from build123d import *

# Parameters (mm, degrees)
SKETCH1_W           = 88.9
SKETCH1_H           = 203.2
BOSS_EXTRUDE1_DEPTH = 6.35
SKETCH2_R           = 3
SKETCH2_R_2         = 2.75
SKETCH2_R_3         = 12.7
CUT_EXTRUDE1_DEPTH  = 7.35


with BuildPart() as part:
    # Sketch1 → Boss-Extrude1 (new body)
    with BuildSketch(Plane(origin=(0, 0, 0), x_dir=(1, 0, 0), z_dir=(0, 1, 0))):
        with Locations((44.45, 101.6)):
            Rectangle(SKETCH1_W, SKETCH1_H)
    extrude(amount=BOSS_EXTRUDE1_DEPTH)

    # Sketch2 → Cut-Extrude1 (cut, through all)
    with BuildSketch(Plane.XZ):
        with Locations((20.6375, -7.913544442)):
            Circle(SKETCH2_R)
        with Locations((68.2625, -7.913544442)):
            Circle(SKETCH2_R)
        with Locations((44.45, -112.75)):
            Circle(SKETCH2_R_2)
        with Locations((8.95, -184.15)):
            Circle(SKETCH2_R_2)
        with Locations((79.95, -184.15)):
            Circle(SKETCH2_R_2)
        with Locations((44.45, -138.15)):
            Circle(SKETCH2_R_3)
    extrude(amount=-CUT_EXTRUDE1_DEPTH, mode=Mode.SUBTRACT)


solid = part.part
Read the model definition and answer for the solid it produces. Units are mm, in the model's axes. Coordinates: 2 decimals unless noted, no trailing zeros. Loops run counter-clockwise (first coordinate to the right, second up) from the corner with the lowest first, then second, coordinate; pieces in that order, holes last.
Q1. The part is cut by section A-A on z = -184.15. Write down the section's boundary in (x, y).
Q2. The mould has two halves that part along Z. Classify faces 1 (the face through (44, 3, -203.2)), 2 (the face through (44, 3, 0)), 3 (the face through (65.265, 3.131, -7.782)), 4 (the face through (0, 3, -100)): +Z half, -Z half, draft (parallel to the pull), parting line (faces both ways), or undercut.
Q3. Consider probe 1 along Z at (x, y) = (44.45, 2); probe 2 along Z at (x, y) = (79.95, 1.75); probe 3 along Z at (x, y) = (11, 0.5). Determine where each line is inside the solid, lowest interval first.
Q4. The part is cut by section C-C on x = 79.95. Write down the section's boundary in (y, z), and give its area (3 significant figures).
Q5. The part is cut by section B-B on z = -112.75. Write down the section's boundary in (x, y).
Q6. The part is cut by section D-D on x = 44.45. Write down the section's boundary in (y, z).
Q7. This flat-tipped pin is pushed along its axis until it touches: pin 1 Ø1 at (x, y) = (61.5, 4) entering from +Z. Where does it stop, or does it pass through?
Results below:
1. outline: (0, 0) - (6.2, 0) - (6.2, 6.35) - (0, 6.35) - close; (11.7, 0) - (77.2, 0) - (77.2, 6.35) - (11.7, 6.35) - close; (82.7, 0) - (88.9, 0) - (88.9, 6.35) - (82.7, 6.35) - close
2. face 1: -Z half
2. face 2: +Z half
2. face 3: undercut
2. face 4: draft
3. probe 1: z = -203.2 to -150.85, -125.45 to -115.5, -110 to 0
3. probe 2: z = -203.2 to -186.9, -181.4 to 0
3. probe 3: z = -203.2 to -185.98, -182.32 to 0
4. outline: (0, -203.2) - (6.35, -203.2) - (6.35, -186.9) - (0, -186.9) - close; (0, -181.4) - (6.35, -181.4) - (6.35, 0) - (0, 0) - close
4. area: 1,260 mm2
5. outline: (0, 0) - (41.7, 0) - (41.7, 6.35) - (0, 6.35) - close; (47.2, 0) - (88.9, 0) - (88.9, 6.35) - (47.2, 6.35) - close
6. outline: (0, -203.2) - (6.35, -203.2) - (6.35, -150.85) - (0, -150.85) - close; (0, -125.45) - (6.35, -125.45) - (6.35, -115.5) - (0, -115.5) - close; (0, -110) - (6.35, -110) - (6.35, 0) - (0, 0) - close
7. pin 1: stops at z = 0
